```python
from build123d import *

# Parameters (mm, degrees)
ESBO_O1_W                = 60
ESBO_O1_H                = 40
RESSALTO_EXTRUS_O1_DEPTH = 1.5
ESBO_O2_R                = 1
CORTE_EXTRUS_O1_DEPTH    = 2.5
ESBO_O3_W                = 1.5
ESBO_O3_H                = 18
RESSALTO_EXTRUS_O2_DEPTH = 20


with BuildPart() as part:
    # Esboço1 → Ressalto-extrusão1 (new body)
    with BuildSketch(Plane.XY):
        Rectangle(ESBO_O1_W, ESBO_O1_H)
    extrude(amount=RESSALTO_EXTRUS_O1_DEPTH)

    # Esboço2 → Corte-extrusão1 (cut, through all)
    with BuildSketch(Plane.XY.offset(1.5)):
        with Locations((-28, 18)):
            Circle(ESBO_O2_R)
        with Locations((28, 18)):
            Circle(ESBO_O2_R)
        with Locations((28, -18)):
            Circle(ESBO_O2_R)
        with Locations((-28, -18)):
            Circle(ESBO_O2_R)
    extrude(amount=-CORTE_EXTRUS_O1_DEPTH, mode=Mode.SUBTRACT)

    # Esboço3 → Ressalto-extrusão2 (add)
    with BuildSketch(Plane.XY.offset(1.5)):
        with Locations((3.833169049, -2.364388559)):
            Rectangle(ESBO_O3_W, ESBO_O3_H)
    extrude(amount=RESSALTO_EXTRUS_O2_DEPTH)


solid = part.part
```
Geometry check sheet. Reference: the model listing, model coordinates, mm. A direction names the side the tool comes from. Coordinates: 2 decimals unless noted, no trailing zeros. Loops run counter-clockwise (first coordinate to the right, second up) from the corner with the lowest first, then second, coordinate; pieces in that order, holes last. Notation, with made-up numbers: (62.25, 62.5) - (101.25, 62.5) arc R18 ccw to (101.25, 88.5) - close; hole circle Ø7 at (70.5, 73). An arc over 180 degrees is marked (long way). One line per item, written item: value. Start each with the question number.
(1) Mould release check, pull along X, two halves, no side actions. Record for faces 5 (the cylindrical face through (-28, -19, 1)), 6 (the flat face through (30, 0, 1)), 7 (the flat face through (4, -11.364, 11)): released by +X, released by -X, zero draft, split by the parting line, or undercut.
(2) Cross-section at B-B on y = 18. Enter the section's corners in (x, z).
(3) Depth check by flat-ended pin: P1, Ø3, axis at x = 28, y = -18, coming from the +Z side; P2, Ø5.5, axis at y = -5.5, z = 16.5, coming from the +X side; P3, Ø0.5, axis at x = 4, z = 10, coming from the +Y side. Enter the tip coordinate at first touch or a pass-through.
(4) Cross-section at D-D on x = -22. Enter the section's corners in (y, z), plus the area to 3 significant figures.
(5) Material ranges on line 1 (Y direction, x = -28, z = 0.8); line 2 (Z direction, x = -11, y = 12); line 3 (X direction, y = -10, z = 12.5), recorded low to high. Write a range as [from, to].
(6) Cross-section at A-A on x = -28. Enter the section's corners in (y, z), plus the area to 3 significant figures.
(7) Cross-section at C-C on z = 8.5. Enter the section's corners in (x, y).
(8) Tool access check on faces 1 (the flat face through (4.583, -2, 11)), 2 (the flat face through (3.083, -2, 11)), 3 (the cylindrical face through (-28, 17, 1)), 4 (the flat face through (4, 6.636, 11)). Record the directions out of +Z, -Z, +X, -X, +Y, -Y that give a thin tool (end or side, any length) a straight path to the whole face; none if there is none.
Results below:
1. face 5: undercut
1. face 6: released by +X
1. face 7: zero draft
2. outline: (-30, 0) - (-29, 0) - (-29, 1.5) - (-30, 1.5) - close; (-27, 0) - (27, 0) - (27, 1.5) - (-27, 1.5) - close; (29, 0) - (30, 0) - (30, 1.5) - (29, 1.5) - close
3. P1: stops at z = 1.5
3. P2: stops at x = 4.58
3. P3: stops at y = 6.64
4. outline: (-20, 0) - (20, 0) - (20, 1.5) - (-20, 1.5) - close
4. area: 60.0 mm2
5. line 1: y = [-20, -19], [-17, 17], [19, 20]
5. line 2: z = [0, 1.5]
5. line 3: x = [3.08, 4.58]
6. outline: (-20, 0) - (-19, 0) - (-19, 1.5) - (-20, 1.5) - close; (-17, 0) - (17, 0) - (17, 1.5) - (-17, 1.5) - close; (19, 0) - (20, 0) - (20, 1.5) - (19, 1.5) - close
6. area: 54.0 mm2
7. outline: (3.08, -11.36) - (4.58, -11.36) - (4.58, 6.64) - (3.08, 6.64) - close
8. face 1: +Z, +X, +Y, -Y
8. face 2: +Z, -X, +Y, -Y
8. face 3: +Z, -Z
8. face 4: +Z, +X, -X, +Y
